Input: dimensioned drawing with shaded views. Units: mm. Origin: part minimum x, y, z. Coordinates: 2 decimals unless noted, no trailing zeros. Order: outer loops, then holes, each group sorted by start corner. A loop starts at its lowest first (then second) coordinate and runs counter-clockwise, first axis right, second up. Notation, with made-up numbers: (-30, -6.75) - (1, -6.75) arc R32 cw to (1, 28.25) - close; hole circle Ø5 at (-24, 7.25). An arc over 180 degrees is marked (long way). One line per question, with ' | ' between items. Start each with the question number.
(1) Contact query for flat-ended pins moving along their axis: P1, Ø5, axis at x = 351.5, y = 293.5, coming from the -Z side; P2, Ø11, axis at x = 83, y = 360, coming from the +Z side. Output: stop coordinate, or through.
(2) Section B-B (z = 35). Count the separate pieces of the cut face and the enclosed holes in it, then the cut area to 3 significant figures.
(3) Section C-C (y = 360). Return the cut outline in (x, z), then the cut area to 3 significant figures.
(4) Line query: line 1 along Y through (x, z) = (513, 21.5); line 2 along Y through (x, z) = (36, 35). Output: solid intervals per line, ascending.
(5) Section A-A (x = 36). Return the cut outline in (y, z).
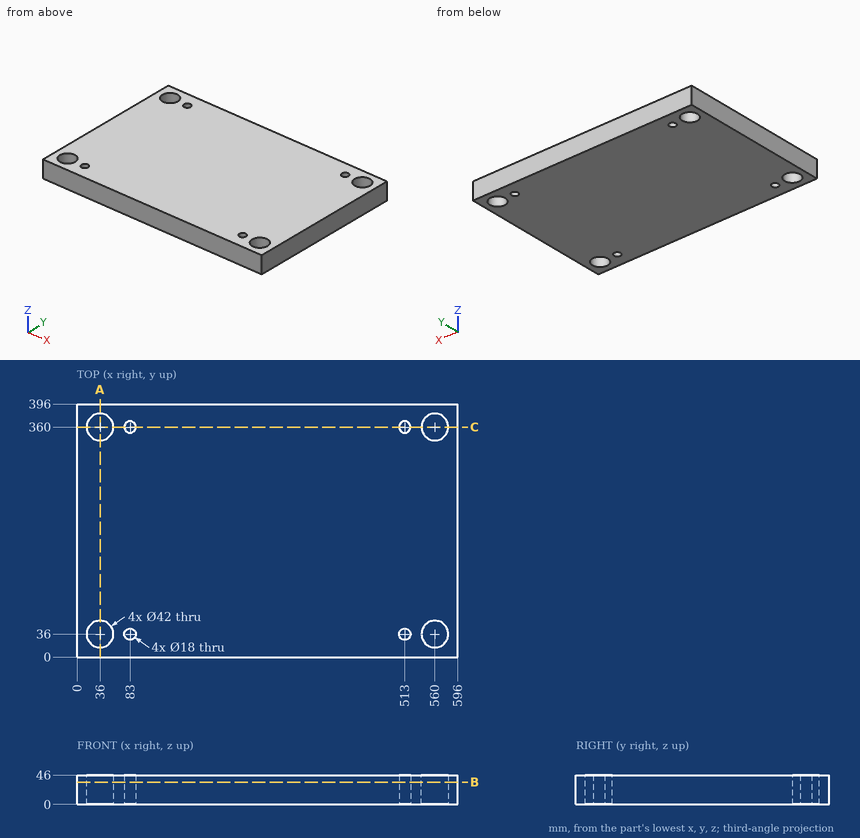
Response values:
1) P1: stops at z = 0 | P2: passes through
2) separate pieces: 1 | enclosed holes: 8 | area: 229,000 mm²
3) outline: (0, 0) - (15, 0) - (15, 46) - (0, 46) - close; (57, 0) - (74, 0) - (74, 46) - (57, 46) - close; (92, 0) - (504, 0) - (504, 46) - (92, 46) - close; (522, 0) - (539, 0) - (539, 46) - (522, 46) - close; (581, 0) - (596, 0) - (596, 46) - (581, 46) - close | area: 21,900 mm²
4) line 1: y = 0 to 27, 45 to 351, 369 to 396 | line 2: y = 0 to 15, 57 to 339, 381 to 396
5) outline: (0, 0) - (15, 0) - (15, 46) - (0, 46) - close; (57, 0) - (339, 0) - (339, 46) - (57, 46) - close; (381, 0) - (396, 0) - (396, 46) - (381, 46) - close
